Here's how the part is built. I have some questions about the finished solid (model axes, mm). Face numbers are marked on the shaded views. A direction names the side the tool comes from. Round coordinates to 2 decimals unless told otherwise and drop trailing zeros. Order: outer loops, then holes, each group sorted by start corner. A loop starts at its lowest first (then second) coordinate and runs counter-clockwise, first axis right, second up.
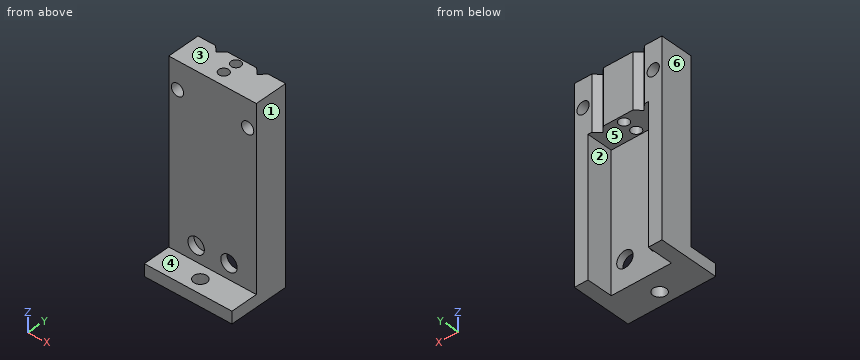
Autodesk Inventor part; units mm, degrees
ref_plane "YZ Plane" through (0, 0, 0) normal (1, 0, 0) x (0, 1, 0)
ref_plane "XZ Plane" through (0, 0, 0) normal (0, 1, 0) x (-1, 0, 0)
ref_plane "XY Plane" through (0, 0, 0) normal (0, 0, 1) x (1, 0, 0)
sketch "Sketch1" plane through (0, 0, 0) normal (0, 0, 1) x (1, 0, 0)
  line L0 (-10.16, 3.81) -> (10.16, 3.81)
  line L1 (10.16, 3.81) -> (10.16, -3.81)
  line L2 (10.16, -3.81) -> (-10.16, -3.81)
  line L3 (-10.16, -3.81) -> (-10.16, 3.81)
  point P0 (0, 0)
  dimension "d0" = 20.32
  dimension "d1" = 7.62
  dimension "d2" = 3.81
  dimension "d3" = 10.16
extrude "Extrusion1" add sketch "Sketch1" against normal blind 12.7
sketch "Sketch2" plane through (0, 0, 0) normal (0, 0, 1) x (1, 0, 0)
  line L0 (-10.16, 3.81) -> (10.16, 3.81)
  circle A0 centre (0, 2.286) radius 1.143
  circle A1 centre (0, -0.889) radius 1.143
  circle A2 centre (-4.7625, 3.81) radius 0.9525
  circle A3 centre (4.7625, 3.81) radius 0.9525
  line L1 (-6.1095, 3.81) -> (-3.5541, 1.2546)
  line L2 (-3.4155, 3.81) -> (-5.4913, 1.7342)
  line L3 (3.4155, 3.81) -> (5.9385, 1.2869)
  line L4 (4.5051, 2.2056) -> (6.1095, 3.81)
  point P0 (0, 0)
  point P1 (-4.7625, 2.463)
  point P2 (4.7625, 2.463)
  dimension "d6" = 2.286
  dimension "d7" = 2.286
  dimension "d8" = 1.524
  dimension "d9" = 3.175
  dimension "d10" = 1.905
  dimension "d11" = 1.905
  dimension "d12" = 0
  dimension "d13" = 0
  dimension "d14" = 9.525
  dimension "d15" = 4.7625
  dimension "d16" = 45
  dimension "d17" = 45
  dimension "d18" = 45
  dimension "d19" = 45
extrude "Extrusion3" cut sketch "Sketch2" against normal blind 12.7 contours L0 A3 L3 | A2 L0 | L0 L2 A2 | A2 L1 L0 | L2 L1 A2 | L0 A3 | A3 L4 L3 | L0 L4 A3 | A0 | A1 picked at (-4.7051, 3.27) picked at (4.6576, 3.5103)
sketch "Sketch3" plane through (-10.16, 3.81, 0) normal (0, 1, 0) x (1, 0, 0)
  line L0 (4.0505, 12.7) -> (0, 12.7)
  line L1 (0, 0) -> (0, 12.7)
  line L2 (0, 0) -> (4.0505, 0)
  circle A0 centre (2.0252, 6.35) radius 1.4224
  point P0 (10.16, 0)
  dimension "d24" = 2.8448
  dimension "d25" = 6.35
  dimension "d26" = 12.7
  dimension "d31" = 4.0505
  dimension "d32" = 2.0252
sketch "Sketch4" plane through (10.16, 3.81, 0) normal (0, 1, 0) x (1, 0, 0)
  line L0 (-4.0505, 0) -> (0, 0)
  line L1 (0, 0) -> (0, 12.7)
  circle A0 centre (-2.0252, 6.35) radius 1.4224
  point P0 (-4.0505, 12.7)
  point P1 (-10.16, 0)
  dimension "d27" = 2.8448
  dimension "d28" = 6.35
  dimension "d29" = 4.0505
  dimension "d30" = 2.0252
extrude "Extrusion4" cut sketch "Sketch3" against normal blind 12.7
extrude "Extrusion5" cut sketch "Sketch4" against normal blind 12.7
sketch "Sketch5" plane through (0, 0, -12.7) normal (0, 0, -1) x (-1, 0, 0)
  line L0 (-10.16, -3.81) -> (-10.16, 3.81)
  line L1 (10.16, -3.81) -> (-10.16, -3.81)
  line L2 (10.16, 3.81) -> (10.16, -3.81)
  line L3 (-10.16, 3.81) -> (-6.985, 3.81)
  line L4 (-6.985, 3.81) -> (-6.985, -3.81)
  line L5 (-6.985, -3.81) -> (-10.16, -3.81)
  line L6 (-10.16, -3.81) -> (-10.16, 3.81)
  line L7 (10.16, 3.81) -> (6.985, 3.81)
  line L8 (6.985, 3.81) -> (6.985, -3.81)
  line L9 (6.985, -3.81) -> (10.16, -3.81)
  line L10 (10.16, -3.81) -> (10.16, 3.81)
  line L11 (-10.16, -2.2225) -> (6.985, -2.2225)
  line L12 (6.985, -2.2225) -> (6.985, -3.81)
  line L13 (6.985, -3.81) -> (-10.16, -3.81)
  line L14 (-10.16, -3.81) -> (-10.16, -2.2225)
  point P0 (0, 0)
  dimension "d37" = 3.175
  dimension "d38" = 3.175
  dimension "d39" = 1.5875
extrude "Extrusion6" add sketch "Sketch5" along normal blind 31.75
thread "Thread1"
thread "Thread2"
sketch "Sketch8" plane through (-10.16, -3.81, 0) normal (0, -1, 0) x (1, 0, 0)
  line L0 (20.32, 0) -> (20.32, -44.45)
  line L1 (0, -44.45) -> (20.32, -44.45)
  line L2 (20.32, -44.45) -> (20.32, -41.656)
  line L3 (20.32, -41.656) -> (0, -41.656)
  line L4 (0, -41.656) -> (0, -44.45)
  point P0 (10.16, 0)
  dimension "d58" = 2.794
extrude "Extrusion9" add sketch "Sketch8" along normal blind 6.35
sketch "Sketch9" plane through (-10.16, -3.81, -41.656) normal (0, 0, 1) x (1, 0, 0)
  line L0 (0, 0) -> (20.32, 0)
  line L1 (0, 0) -> (0, -6.35)
  circle A0 centre (10.16, -3.175) radius 1.524
  point P0 (20.32, -6.35)
  point P1 (10.16, 3.81)
  dimension "d61" = 3.048
  dimension "d62" = 20.32
  dimension "d63" = 6.35
  dimension "d64" = 3.175
  dimension "d65" = 10.16
extrude "Extrusion10" cut sketch "Sketch9" against normal blind 7.62
sketch "Sketch10" plane through (-6.985, -2.2225, -12.7) normal (0, 1, 0) x (1, 0, 0)
  line L0 (13.97, 0) -> (13.97, 31.75)
  line L1 (0, 0) -> (0, 31.75)
  line L2 (13.97, 0) -> (0, 0)
  circle A0 centre (3.175, 25.4) radius 1.905
  circle A1 centre (10.795, 25.4) radius 1.905
  point P0 (6.985, -12.7)
  dimension "d68" = 3.81
  dimension "d69" = 3.81
  dimension "d70" = 3.175
  dimension "d71" = 3.175
  dimension "d72" = 25.4
  dimension "d73" = 25.4
extrude "Extrusion11" cut sketch "Sketch10" against normal blind 7.62
equation "\"d7\" = d6"
equation "\"d25\" = 0.5 * d26"
equation "\"d32\" = 0.5 * d31"
equation "\"d28\" = d25"
equation "\"d30\" = 0.5 * d29"
equation "\"d38\" = d37"
equation "\"d64\" = 0.5 * d63"
equation "\"d65\" = 0.5 * d62"
equation "\"d73\" = d72"
properties part number "lickport_Holder_small"
1. If we section it at D-D, the plane y = -7.5: Write out the boundary of the cut face in (x, z).
Evaluation:
outline: (-10.16, -44.45) - (-1.43, -44.45) - (-1.43, -41.66) - (-10.16, -41.66) - close; (1.43, -44.45) - (10.16, -44.45) - (10.16, -41.66) - (1.43, -41.66) - close
2. I'm going to push flat-ended pins straight in: P1, Ø2, axis at x = -4.5, y = -8.5, coming from the +Z side; P2, Ø3.5, axis at x = 8.13, z = -6.35, coming from the -Y side; P3, Ø3, axis at x = 0, y = 0, coming from the -Z side. Where does each tip first touch, or does it pass through?
Evaluation:
P1: stops at z = -41.66
P2: stops at y = -3.81
P3: stops at z = -12.7
3. On a 3-axis mill with a long thin cutter (end or side, diameter ignored), from which of +Z, -Z, +X, -X, +Y, -Y can I reach the whole of each face in a straight line? I mean the marked faces 4, 5 and 6. Say none if no direction works.
Evaluation:
face 4: +Z, +X, -X, -Y
face 5: -Z, +Y
face 6: +Z, -Z, -X, +Y, -Y
4. I need wall thicknesses on probe 1 along X at (y, z) = (-2.6, -38.1) (3 decimals); probe 2 along Y at (x, z) = (0, -9.5); probe 3 along X at (y, z) = (-0.75, -6.35). Which ranges of each line are inside material? Lowest first, please.
Evaluation:
probe 1: x = -10.16 to -5.715, -1.905 to 1.905, 5.715 to 10.16
probe 2: y = -3.81 to -2.03, 0.25 to 1.14, 3.43 to 3.81
probe 3: x = -10.16 to -9.56, -6.71 to -1.13, 1.13 to 6.71, 9.56 to 10.16
5. If we section it at B-B, the plane x = -2.5: Write out the boundary of the cut face in (y, z), and give its area (3 significant figures).
Evaluation:
outline: (-10.16, -44.45) - (-2.22, -44.45) - (-2.22, -39.48) - (-3.81, -39.48) - (-3.81, -41.66) - (-10.16, -41.66) - close; (-3.81, -36.72) - (-2.22, -36.72) - (-2.22, -12.7) - (3.81, -12.7) - (3.81, 0) - (-3.81, 0) - close
area: 161 mm2
6. If we section it at C-C, the plane z = -6.35: Write out the boundary of the cut face in (x, y), and give its area (3 significant figures).
Evaluation:
outline: (-10.16, -3.81) - (-9.56, -3.81) - (-9.56, 3.81) - (-10.16, 3.81) - close; (-6.71, -3.81) - (6.71, -3.81) - (6.71, 3.81) - (6.11, 3.81) - (4.76, 2.46) - (3.42, 3.81) - (-3.42, 3.81) - (-4.76, 2.46) - (-6.11, 3.81) - (-6.71, 3.81) - close; (9.56, -3.81) - (10.16, -3.81) - (10.16, 3.81) - (9.56, 3.81) - close; hole circle Ø2.29 at (0, -0.89); hole circle Ø2.29 at (0, 2.29)
area: 99.6 mm2
7. If we section it at A-A, the plane z = -38.1: Write out the boundary of the cut face in (x, y) (1 decimal).
Evaluation:
outline: (-10.2, -3.8) - (-5.7, -3.8) - (-5.7, -2.2) - (-7, -2.2) - (-7, 3.8) - (-10.2, 3.8) - close; (-1.9, -3.8) - (1.9, -3.8) - (1.9, -2.2) - (-1.9, -2.2) - close; (5.7, -3.8) - (10.2, -3.8) - (10.2, 3.8) - (7, 3.8) - (7, -2.2) - (5.7, -2.2) - close
8. If we mould it in two halves opening along X, with no side actions, what happens to the marked faces 1, 2 and 3? For each: released by +X, released by -X, zero draft, split by the parting line, or undercut.
Evaluation:
face 1: released by +X
face 2: undercut
face 3: zero draft
